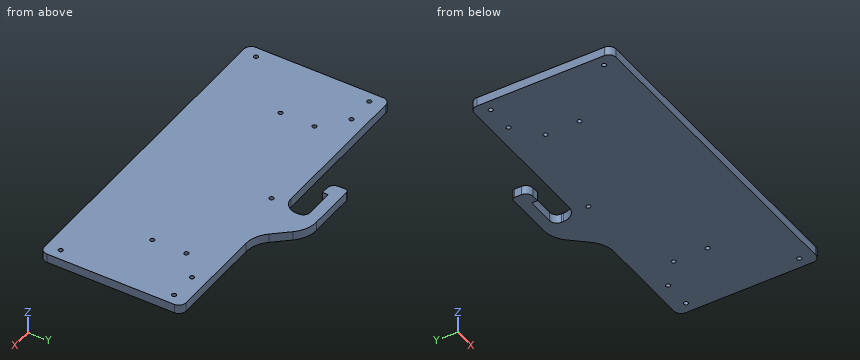
from build123d import *

# Parameters (mm, degrees)
SKETCH1_W           = 233.2
SKETCH1_H           = 100
SKETCH1_R           = 1.55
BOSS_EXTRUDE1_DEPTH = 6.35
FILLET1_R           = 5
SKETCH2_R           = 1.55
CUT_EXTRUDE1_DEPTH  = 6.35
SKETCH3_W           = 10
SKETCH3_H           = 12.7
BOSS_EXTRUDE2_DEPTH = 6.35
FILLET2_R           = 5
FILLET3_R           = 10
FILLET4_R           = 2
FILLET5_R           = 20
FILLET6_R           = 5


with BuildPart() as part:
    # Sketch1 → Boss-Extrude1 (new body)
    with BuildSketch(Plane.XY):
        with Locations((116.6, -50)):
            Rectangle(SKETCH1_W, SKETCH1_H)
        with Locations((7.5, -10)):
            Circle(SKETCH1_R, mode=Mode.SUBTRACT)
        with Locations((225.7, -10)):
            Circle(SKETCH1_R, mode=Mode.SUBTRACT)
        with Locations((7.5, -90)):
            Circle(SKETCH1_R, mode=Mode.SUBTRACT)
        with Locations((225.7, -90)):
            Circle(SKETCH1_R, mode=Mode.SUBTRACT)
        with Locations((27.5, -10)):
            Circle(SKETCH1_R, mode=Mode.SUBTRACT)
        with Locations((205.7, -10)):
            Circle(SKETCH1_R, mode=Mode.SUBTRACT)
        with Locations((116.6, -10)):
            Circle(SKETCH1_R, mode=Mode.SUBTRACT)
    extrude(amount=BOSS_EXTRUDE1_DEPTH)

    # Fillet1
    fillet1_edges = [part.edges().sort_by_distance(p)[0] for p in [
        (233.2, -100, 3.175),
        (0, -100, 3.175),
        (0, 0, 3.175),
        (233.2, 0, 3.175),
    ]]
    fillet(fillet1_edges, radius=FILLET1_R)

    # Sketch2 → Cut-Extrude1 (cut)
    with BuildSketch(Plane.XY.offset(6.35)):
        with Locations((45, -25)):
            Circle(SKETCH2_R)
        with Locations((45, -49)):
            Circle(SKETCH2_R)
        with Locations((188.2, -49)):
            Circle(SKETCH2_R)
        with Locations((188.2, -25)):
            Circle(SKETCH2_R)
    extrude(amount=-CUT_EXTRUDE1_DEPTH, mode=Mode.SUBTRACT)

    # Sketch3 → Boss-Extrude2 (add)
    with BuildSketch(Plane.XY.offset(6.35)):
        with Locations((125.723568259, 6.35)):
            Rectangle(SKETCH3_W, SKETCH3_H)
        Polygon((120.723568259, 16.7), (120.723568259, 12.7), (130.723568259, 12.7), (130.723568259, 24.7), (85.723568259, 24.7), (85.723568259, 12.7), (95.723568259, 12.7), (95.723568259, 16.7), align=None)
        Polygon((130.723568259, 12.7), (130.723568259, 0), (152.313568259, 0), (130.723568259, 24.7), align=None)
    extrude(amount=-BOSS_EXTRUDE2_DEPTH)

    # Fillet2
    fillet2_edges = [part.edges().sort_by_distance(p)[0] for p in [
        (85.723568259, 12.7, 3.175),
    ]]
    fillet(fillet2_edges, radius=FILLET2_R)

    # Fillet3
    fillet3_edges = [part.edges().sort_by_distance(p)[0] for p in [
        (120.723568259, 0, 3.175),
    ]]
    fillet(fillet3_edges, radius=FILLET3_R)

    # Fillet4
    fillet4_edges = [part.edges().sort_by_distance(p)[0] for p in [
        (85.723568259, 24.7, 3.175),
    ]]
    fillet(fillet4_edges, radius=FILLET4_R)

    # Fillet5
    fillet5_edges = [part.edges().sort_by_distance(p)[0] for p in [
        (130.723568259, 24.7, 3.175),
        (152.313568259, 0, 3.175),
    ]]
    fillet(fillet5_edges, radius=FILLET5_R)

    # Fillet6
    fillet6_edges = [part.edges().sort_by_distance(p)[0] for p in [
        (120.723568259, 16.7, 3.175),
    ]]
    fillet(fillet6_edges, radius=FILLET6_R)


solid = part.part
Work out the finished part from the listing and answer in its coordinate system (mm). Coordinates: 2 decimals unless noted, no trailing zeros. Write each loop counter-clockwise with the first axis right and the second up, starting at its lowest first coordinate (ties: lowest second). Pieces come first, ordered by that corner, then holes. Notation, with made-up numbers: M 36.25,63 L 70.25,63 A22 cw 70.25,74 Z; hole C 24,88.5 d3. An arc over 180 degrees is marked long. Write item = value, one per line.
1. Straight lines are drawn through the part: line 1 (Y direction, x = 7.5, z = 2.5); line 2 (Y direction, x = 45, z = 2.5); line 3 (Y direction, x = 27.5, z = 4). For each, find the intervals that lie inside material, in ascending order. Write a range as from..to.
Solution:
line_1 = -100..-91.55, -88.45..-11.55, -8.45..0
line_2 = -100..-50.55, -47.45..-26.55, -23.45..0
line_3 = -100..-11.55, -8.45..0
2. A flat-ended cylindrical pin translates along its axis: pin 1 (3 mm diameter, centred on x = 34.5, z = 4.5, fed in from +Y). Find the tip coordinate at first contact, or state that the pin passes through.
Solution:
pin_1 = 0
3. The part is cut by section B-B (x = 40.5). Determine the outline of the cut face in (y, z), then the cut area to 3 significant figures.
Solution:
outline = M -100,0 L 0,0 L 0,6.35 L -100,6.35 Z
area = 635 mm2
4. The part is cut by section A-A (z = 4.75). State how many separate pieces and enclosed holes the cut face has, then the cut area to 3 significant figures.
Solution:
separate_pieces = 1
enclosed_holes = 11
area = 24,100 mm2
5. The part is cut by section C-C (x = 143). Determine the outline of the cut face in (y, z), then the cut area to 3 significant figures.
Solution:
outline = M -100,0 L 10.66,0 L 10.66,6.35 L -100,6.35 Z
area = 703 mm2
